```python
from build123d import *

# Parameters (mm, degrees)
SKETCH1_R           = 4.7625
EXTRUDE1_DEPTH      = 19.05
SKETCH2_R           = 6.477
EXTRUDE2_DEPTH      = 3.302
CHAMFER1_SIZE       = 0.6604
EXTRUDE3_DEPTH      = 25.156054355
EXTRUDE3_DEPTH_BACK = 25.156054355
SKETCH3_R           = 1.984375
CHAMFER2_SIZE       = 0.47625


with BuildPart() as part:
    # Sketch1 → Extrude1 (new, symmetric)
    with BuildSketch(Plane.XY):
        with Locations(Location((0, 0, 0), (0, 0, 180))):
            Circle(SKETCH1_R)
    extrude(amount=EXTRUDE1_DEPTH, both=True)

    # Sketch2 → Extrude2 (add)
    with BuildSketch(Plane.XY.offset(19.05)):
        with Locations(Location((0, 0, 0), (0, 0, 180))):
            Circle(SKETCH2_R)
    extrude(amount=EXTRUDE2_DEPTH)

    # Chamfer1
    chamfer1_edges = [part.edges().sort_by_distance(p)[0] for p in [
        (6.477, 0, 22.352),
    ]]
    chamfer(chamfer1_edges, length=CHAMFER1_SIZE)

    # Sketch3 → Extrude3 (cut, two sides: drawn at the far end of the back side and taken through both)
    with BuildSketch(Plane(origin=(0, 0, 0), x_dir=(0, 0, -1), z_dir=(1, 0, 0)).offset(-EXTRUDE3_DEPTH_BACK)):
        with Locations(Location((14.684375, 0, 0), (0, 0, 180.000000002))):
            Circle(SKETCH3_R)
    extrude(amount=EXTRUDE3_DEPTH + EXTRUDE3_DEPTH_BACK, mode=Mode.SUBTRACT)

    # Chamfer2
    chamfer2_edges = [part.edges().sort_by_distance(p)[0] for p in [
        (4.7625, 0, -19.05),
    ]]
    chamfer(chamfer2_edges, length=CHAMFER2_SIZE)


solid = part.part
```
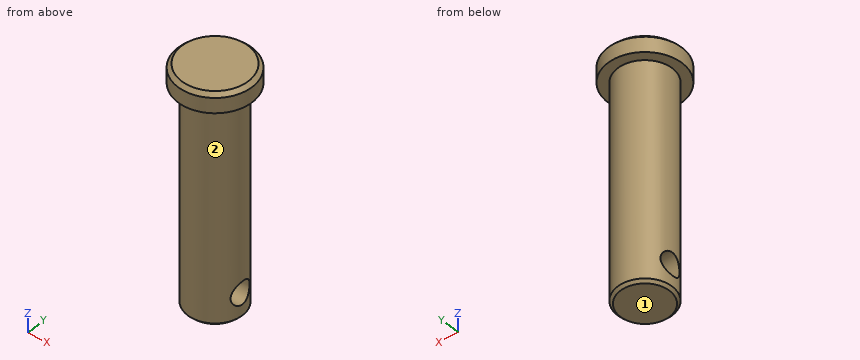
Part model, mm, in its own coordinate system. Face numbers are marked on the shaded views. A direction names the side the tool comes from. Round coordinates to 2 decimals unless told otherwise and drop trailing zeros. Order: outer loops, then holes, each group sorted by start corner. A loop starts at its lowest first (then second) coordinate and runs counter-clockwise, first axis right, second up. Notation, with made-up numbers: M 64,67 L 106,67 A17 ccw 106,81 Z; hole C -1.5,66 d3. An arc over 180 degrees is marked long. Put each result on its own line as item: value. Start each with the question number.
1. Tool access for the marked faces 1 and 2: list every direction of +Z, -Z, +X, -X, +Y, -Y with a clear straight run to the whole face (end or side of a thin tool).
2. Slice it at A-A on y = 0. List the corners of the cut face in (x, z), then the cut area to 3 significant figures.
3. Drop flat-ended pins along their axis: pin 1 (6 mm diameter, centred on y = -2, z = 17, fed in from +X); pin 2 (1.5 mm diameter, centred on x = 3, z = 7, fed in from -Y); pin 3 (3 mm diameter, centred on y = 0, z = -14.68, fed in from +X); pin 4 (5 mm diameter, centred on y = 3, z = 14, fed in from -X). Give the stop position or say it passes through.
4. Drill centre lines: probe 1 along Z at (x, y) = (-0.75, 0); probe 2 along Y at (x, z) = (0, -4); probe 3 along Y at (x, z) = (3.5, -14). Where is each one in solid material? Low to high. Write a range as [from, to].
5. Slice it at B-B on x = 0. List the corners of the cut face in (y, z), then the cut area to 3 significant figures.
6. Slice it at C-C on z = 14. List the corners of the cut face in (x, y) (1 decimal), then the cut area to 3 significant figures.
Findings:
1. face 1: -Z, +X, -X, +Y, -Y
1. face 2: -Z
2. outline: M -6.48,19.05 L -4.76,19.05 L -4.76,-12.7 L 4.76,-12.7 L 4.76,19.05 L 6.48,19.05 L 6.48,21.69 L 5.82,22.35 L -5.82,22.35 L -6.48,21.69 Z; M -4.76,-18.57 L -4.29,-19.05 L 4.29,-19.05 L 4.76,-18.57 L 4.76,-16.67 L -4.76,-16.67 Z
2. area: 367 mm2
3. pin 1: x = 6.48
3. pin 2: y = -4.2
3. pin 3: through
3. pin 4: x = -4.74
4. probe 1: [-19.05, -16.67], [-12.7, 22.35]
4. probe 2: [-4.76, 4.76]
4. probe 3: [-3.23, -1.86], [1.86, 3.23]
5. outline: M -6.48,19.05 L -4.76,19.05 L -4.76,-18.57 L -4.29,-19.05 L 4.29,-19.05 L 4.76,-18.57 L 4.76,19.05 L 6.48,19.05 L 6.48,21.69 L 5.82,22.35 L -5.82,22.35 L -6.48,21.69 Z; hole C 0,-14.68 d3.97
5. area: 393 mm2
6. outline: C 0,0 d9.5
6. area: 71.3 mm2
